```python
from build123d import *

# Parameters (mm, degrees)
ESQUISSE1_W                 = 200
ESQUISSE1_H                 = 200
BOSS_EXTRU_PAROIE_DEPTH     = 4
BOSS_EXTRU_BORDS_DEPTH      = 8
BOSS_EXTRU_GLISSIERES_DEPTH = 5
CONG_1_R                    = 1
ESQUISSE8_W                 = 1.8
ESQUISSE8_H                 = 180
ENL_V_MAT_EXTRU_6_DEPTH     = 9
ESQUISSE5_R                 = 1.6
ENL_V_MAT_EXTRU_2_DEPTH     = 10
ESQUISSE6_R                 = 1.6
ENL_V_MAT_EXTRU_3_DEPTH     = 10
ESQUISSE7_R                 = 1.6
ENL_V_MAT_EXTRU_4_DEPTH     = 10
ESQUISSE10_R                = 1.6
ENL_V_MAT_EXTRU_8_DEPTH     = 10
ESQUISSE11_W                = 113.303164178
ESQUISSE11_H                = 6
ENL_V_MAT_EXTRU_9_DEPTH     = 6
ESQUISSE9_R                 = 1.6
ENL_V_MAT_EXTRU_10_DEPTH    = 10


with BuildPart() as part:
    # Esquisse1 → Boss.-Extru. Paroie (new body)
    with BuildSketch(Plane.XY):
        with Locations((100, 100)):
            Rectangle(ESQUISSE1_W, ESQUISSE1_H)
    extrude(amount=BOSS_EXTRU_PAROIE_DEPTH)

    # Esquisse4 → Boss.-Extru. Bords (add)
    with BuildSketch(Plane.XY.offset(4)):
        Polygon((3, 3), (9, 3), (9, 184), (191, 184), (191, 3), (197, 3), (197, 197), (191, 197), (191, 190), (9, 190), (9, 197), (3, 197), align=None)
    extrude(amount=BOSS_EXTRU_BORDS_DEPTH)

    # Esquisse2 → Boss.-Extru. Glissieres (add)
    with BuildSketch(Plane.XY.offset(4)):
        with BuildLine():
            Line((47, 180), (53, 180))
            ThreePointArc((53, 180), (54.414213562, 179.414213562), (55, 178))
            Line((55, 178), (55, 12))
            ThreePointArc((55, 12), (54.414213562, 10.585786438), (53, 10))
            Line((53, 10), (47, 10))
            ThreePointArc((47, 10), (45.585786438, 10.585786438), (45, 12))
            Line((45, 12), (45, 178))
            ThreePointArc((45, 178), (45.585786438, 179.414213562), (47, 180))
        make_face()
        with BuildLine():
            Line((97, 180), (103, 180))
            ThreePointArc((103, 180), (104.414213562, 179.414213562), (105, 178))
            Line((105, 178), (105, 12))
            ThreePointArc((105, 12), (104.414213562, 10.585786438), (103, 10))
            Line((103, 10), (97, 10))
            ThreePointArc((97, 10), (95.585786438, 10.585786438), (95, 12))
            Line((95, 12), (95, 178))
            ThreePointArc((95, 178), (95.585786438, 179.414213562), (97, 180))
        make_face()
        with BuildLine():
            Line((147, 180), (153, 180))
            ThreePointArc((153, 180), (154.414213562, 179.414213562), (155, 178))
            Line((155, 178), (155, 12))
            ThreePointArc((155, 12), (154.414213562, 10.585786438), (153, 10))
            Line((153, 10), (147, 10))
            ThreePointArc((147, 10), (145.585786438, 10.585786438), (145, 12))
            Line((145, 12), (145, 178))
            ThreePointArc((145, 178), (145.585786438, 179.414213562), (147, 180))
        make_face()
    extrude(amount=BOSS_EXTRU_GLISSIERES_DEPTH)

    # Congé1
    cong_1_edges = [part.edges().sort_by_distance(p)[0] for p in [
        (200, 100, 4),
        (100, 200, 4),
        (0, 100, 4),
        (100, 0, 4),
    ]]
    fillet(cong_1_edges, radius=CONG_1_R)

    # Esquisse8 → Enlèv. mat.-Extru.6 (cut, through all)
    with BuildSketch(Plane.XY.offset(4)):
        with Locations((100, 85)):
            Rectangle(ESQUISSE8_W, ESQUISSE8_H)
        with Locations((150, 85)):
            Rectangle(ESQUISSE8_W, ESQUISSE8_H)
        with Locations((50, 85)):
            Rectangle(ESQUISSE8_W, ESQUISSE8_H)
    extrude(amount=ENL_V_MAT_EXTRU_6_DEPTH, mode=Mode.SUBTRACT)

    # Esquisse5 → Enlèv. mat.-Extru.2 (cut)
    with BuildSketch(Plane.ZY.offset(-3)):
        with Locations((8, 180)):
            Circle(ESQUISSE5_R)
        with Locations((8, 20)):
            Circle(ESQUISSE5_R)
    extrude(amount=-ENL_V_MAT_EXTRU_2_DEPTH, mode=Mode.SUBTRACT)

    # Esquisse6 → Enlèv. mat.-Extru.3 (cut)
    with BuildSketch(Plane(origin=(197, 0, 0), x_dir=(0, 0, -1), z_dir=(1, 0, 0))):
        with Locations((-8, 180)):
            Circle(ESQUISSE6_R)
        with Locations((-8, 20)):
            Circle(ESQUISSE6_R)
    extrude(amount=-ENL_V_MAT_EXTRU_3_DEPTH, mode=Mode.SUBTRACT)

    # Esquisse7 → Enlèv. mat.-Extru.4 (cut)
    with BuildSketch(Plane.XZ.offset(-184)):
        with Locations((35, 8)):
            Circle(ESQUISSE7_R)
        with Locations((165, 8)):
            Circle(ESQUISSE7_R)
    extrude(amount=-ENL_V_MAT_EXTRU_4_DEPTH, mode=Mode.SUBTRACT)

    # Esquisse10 → Enlèv. mat.-Extru.8 (cut)
    with BuildSketch(Plane(origin=(0, 3, 0), x_dir=(-1, 0, 0), z_dir=(0, -1, 0))):
        with Locations((-194.2, -8)):
            Circle(ESQUISSE10_R)
        with Locations((-5.8, -8)):
            Circle(ESQUISSE10_R)
    extrude(amount=-ENL_V_MAT_EXTRU_8_DEPTH, mode=Mode.SUBTRACT)

    # Esquisse11 → Enlèv. mat.-Extru.9 (cut)
    with BuildSketch(Plane.XY.offset(12)):
        with Locations((100.248809194, 187)):
            Rectangle(ESQUISSE11_W, ESQUISSE11_H)
    extrude(amount=-ENL_V_MAT_EXTRU_9_DEPTH, mode=Mode.SUBTRACT)

    # Esquisse9 → Enlèv. mat.-Extru.10 (cut)
    with BuildSketch(Plane(origin=(0, 197, 0), x_dir=(1, 0, 0), z_dir=(0, 1, 0))):
        with Locations((194.2, -8)):
            Circle(ESQUISSE9_R)
        with Locations((5.8, -8)):
            Circle(ESQUISSE9_R)
    extrude(amount=-ENL_V_MAT_EXTRU_10_DEPTH, mode=Mode.SUBTRACT)


solid = part.part
```
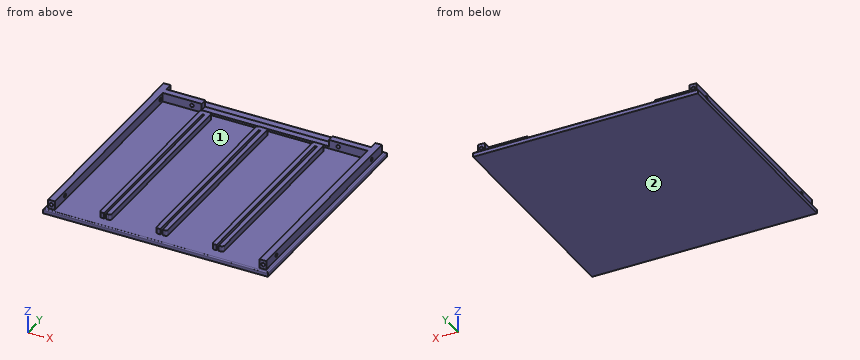
Geometry: final body of the model. Coordinates: model frame, mm. Face numbers are marked on the shaded views. Coordinates: 2 decimals unless noted, no trailing zeros. Order: outer loops, then holes, each group sorted by start corner. A loop starts at its lowest first (then second) coordinate and runs counter-clockwise, first axis right, second up. Notation, with made-up numbers: (77.25, 77.5) - (106.25, 77.5) arc R25 ccw to (106.25, 111.5) - close; hole circle Ø2 at (-31, -24). An arc over 180 degrees is marked (long way). Return JSON: item names as keys, results as strings. Group by question number.
1. Pull-direction query (X, two-part tool) for the marked faces 1 and 2; classes: pulls with the +X half, pulls with the -X half, needs draft (parallel to the pull), parting line crosses it, or undercut.
2. Material intervals for line 1 along Y through (x, z) = (195, 8); line 2 along X through (y, z) = (191, 8); line 3 along Z through (x, y) = (5.8, 191.75), sorted ascending. Write a range as [from, to].
3. Cut plane A-A (x = 92). Output: boundary loops of the cut face in (y, z), plus the area to 3 significant figures.
4. Pin query (flat end, axial travel): pin 1 (4 mm diameter, centred on y = 80.5, z = 7, fed in from +X); pin 2 (3 mm diameter, centred on x = 160, y = 171, fed in from +Z); pin 3 (2.5 mm diameter, centred on y = 85.5, z = 6.5, fed in from -X). Return the tip coordinate at first contact, or that it passes through.
Resolved:
{
 "1": {"face 1": "undercut", "face 2": "needs draft"},
 "2": {"line 1": "y = [13, 18.4], [21.6, 178.4], [181.6, 187]", "line 2": "x = [3, 4.2], [7.4, 9], [191, 192.6], [195.8, 197]", "line 3": "z = [0, 6.4], [9.6, 12]"},
 "3": {"outline": "(0, 0) - (200, 0) - (200, 3) arc R1 ccw to (199, 4) - (190, 4) - (190, 6) - (184, 6) - (184, 4) - (1, 4) arc R1 ccw to (0, 3) - close", "area": "812 mm²"},
 "4": {"pin 1": "stops at x = 197", "pin 2": "stops at z = 4", "pin 3": "stops at x = 3"}
}
